from build123d import *

# Parameters (mm, degrees)
CROQUIS1_R              = 2
SALIENTE_EXTRUIR1_DEPTH = 41
CROQUIS2_R              = 12.55
SALIENTE_EXTRUIR2_DEPTH = 3
CROQUIS3_R              = 2.5
SALIENTE_EXTRUIR3_DEPTH = 19
CHAFL_N1_SIZE           = 1


with BuildPart() as part:
    # Croquis1 → Saliente-Extruir1 (new body)
    with BuildSketch(Plane.XY):
        Polygon((-21, 16), (-16, 21), (16, 21), (21, 16), (21, -16), (16, -21), (-16, -21), (-21, -16), align=None)
        with Locations((12.727922061, 12.727922061)):
            Circle(CROQUIS1_R, mode=Mode.SUBTRACT)
        with Locations((12.727922061, -12.727922061)):
            Circle(CROQUIS1_R, mode=Mode.SUBTRACT)
        with Locations((-12.727922061, -12.727922061)):
            Circle(CROQUIS1_R, mode=Mode.SUBTRACT)
        with Locations((-12.727922061, 12.727922061)):
            Circle(CROQUIS1_R, mode=Mode.SUBTRACT)
    extrude(amount=SALIENTE_EXTRUIR1_DEPTH)

    # Croquis2 → Saliente-Extruir2 (add)
    with BuildSketch(Plane.XY.offset(41)):
        Circle(CROQUIS2_R)
    extrude(amount=SALIENTE_EXTRUIR2_DEPTH)

    # Croquis3 → Saliente-Extruir3 (add)
    with BuildSketch(Plane.XY.offset(44)):
        Circle(CROQUIS3_R)
    extrude(amount=SALIENTE_EXTRUIR3_DEPTH)

    # Chaflán1
    chafl_n1_edges = [part.edges().sort_by_distance(p)[0] for p in [
        (-12.55, 0, 44),
    ]]
    chamfer(chafl_n1_edges, length=CHAFL_N1_SIZE)


solid = part.part
The model under review builds one solid part; all positions refer to its coordinate system, in mm. A direction names the side the tool comes from. Round coordinates to 2 decimals unless told otherwise and drop trailing zeros. Write each loop counter-clockwise with the first axis right and the second up, starting at its lowest first coordinate (ties: lowest second). Pieces come first, ordered by that corner, then holes. Notation, with made-up numbers: (-23.5, 67.5) -> (-11.5, 67.5) arc R21 ccw to (-11.5, 83.5) -> close; hole circle Ø11 at (5, 39.25). An arc over 180 degrees is marked (long way). Answer as a JSON object with one key per item and string values.
1. We need section D-D on z = 48. State the section outline as (x, y) points.
Results found:
{"outline": "circle Ø5 at (0, 0)"}
2. To check wall thickness, follow line 1 along Y through (x, z) = (-12, 8.5); line 2 along X through (y, z) = (13, 17); line 3 along Z through (x, y) = (-4, -18). State the ranges of each line that lie inside material, in increasing order.
Results found:
{"line 1": "y = -21 to -14.59, -10.87 to 10.87, 14.59 to 21", "line 2": "x = -21 to -14.71, -10.75 to 10.75, 14.71 to 21", "line 3": "z = 0 to 41"}
3. We need section A-A on z = 28. State the section outline as (x, y) points, and give its area (3 significant figures).
Results found:
{"outline": "(-21, -16) -> (-16, -21) -> (16, -21) -> (21, -16) -> (21, 16) -> (16, 21) -> (-16, 21) -> (-21, 16) -> close; hole circle Ø4 at (-12.73, -12.73); hole circle Ø4 at (-12.73, 12.73); hole circle Ø4 at (12.73, -12.73); hole circle Ø4 at (12.73, 12.73)", "area": "1,660 mm^2"}
4. We need section B-B on x = 0. State the section outline as (y, z) points, and give its area (3 significant figures).
Results found:
{"outline": "(-21, 0) -> (21, 0) -> (21, 41) -> (12.55, 41) -> (12.55, 43) -> (11.55, 44) -> (2.5, 44) -> (2.5, 63) -> (-2.5, 63) -> (-2.5, 44) -> (-11.55, 44) -> (-12.55, 43) -> (-12.55, 41) -> (-21, 41) -> close", "area": "1,890 mm^2"}
5. Clearance check with flat-ended pins moving along their axes: pin 1 (4 mm diameter, centred on x = 6, y = -4.5, fed in from +Z); pin 2 (3 mm diameter, centred on x = -12.73, y = 12.73, fed in from +Z); pin 3 (4 mm diameter, centred on x = 14, y = -1, fed in from +Z); pin 4 (4.5 mm diameter, centred on x = 12.73, y = -12.73, fed in from +Z). State where each tip first meets the part, or that it passes through.
Results found:
{"pin 1": "stops at z = 44", "pin 2": "passes through", "pin 3": "stops at z = 43.51", "pin 4": "stops at z = 41"}
6. Machinability: for faces 1 (the face through (-19, 18, 20)), 2 (the face through (-0.54, -2.44, 53.37)), which of the approach directions +Z, -Z, +X, -X, +Y, -Y give a long, thin tool a straight path to every point of the face, cutting with its end or side? Answer none if there is none.
Results found:
{"face 1": "+Z, -Z, -X, +Y", "face 2": "+Z"}
7. We need section C-C on y = 18.5. State the section outline as (x, z) points.
Results found:
{"outline": "(-18.5, 0) -> (18.5, 0) -> (18.5, 41) -> (-18.5, 41) -> close"}
